```python
from build123d import *

# Parameters (mm, degrees)
F0_W     = 90
F0_H     = 41.77
F1_DEPTH = 6
F3_DEPTH = 36.63
F4_R     = 3
F5_R     = 1.5
F6_DEPTH = 5


with BuildPart() as f1:
    # F0 (on Front) → F1 (new body, symmetric)
    with BuildSketch(Plane.XZ):
        Rectangle(F0_W, F0_H)
    extrude(amount=F1_DEPTH, both=True)

    # F2 (on face) → F3 (join)
    with BuildSketch(Plane.XY.offset(20.885)):
        with BuildLine():
            Line((-28, 0), (-23, 0))
            ThreePointArc((-23, 0), (-28, 5), (-33, 0))
            Line((-33, 0), (-28, 0))
        make_face()
        with BuildLine():
            ThreePointArc((-33, 0), (-28, -5), (-23, 0))
            Line((-23, 0), (-28, 0))
            Line((-28, 0), (-33, 0))
        make_face()
        with BuildLine():
            Line((-5, 0), (0, 0))
            Line((0, 0), (5, 0))
            ThreePointArc((5, 0), (0, 5), (-5, 0))
        make_face()
        with BuildLine():
            Line((5, 0), (0, 0))
            Line((0, 0), (-5, 0))
            ThreePointArc((-5, 0), (0, -5), (5, 0))
        make_face()
        with BuildLine():
            ThreePointArc((33, 0), (28, 5), (23, 0))
            ThreePointArc((23, 0), (28, -5), (33, 0))
        make_face()
    extrude(amount=F3_DEPTH)

    # F4
    f4_edges = [f1.edges().sort_by_distance(p)[0] for p in [
        (45, -6, 0),
        (45, 6, 0),
        (-45, -6, 0),
        (-45, 6, 0),
    ]]
    fillet(f4_edges, radius=F4_R)

    # F5 (on face) → F6 (join)
    with BuildSketch(Plane.XY.offset(57.515)):
        with Locations((-28, 0)):
            Circle(F5_R)
        Circle(F5_R)
        with Locations((28, 0)):
            Circle(F5_R)
    extrude(amount=F6_DEPTH)


solid = f1.part
```
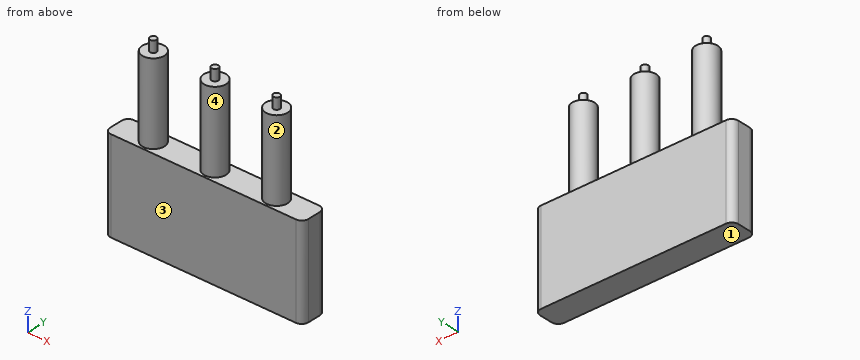
Can you work these out from the model? Positions are in its coordinate system, mm. Face numbers are marked on the shaded views. A direction names the side the tool comes from. Round coordinates to 2 decimals unless told otherwise and drop trailing zeros. Order: outer loops, then holes, each group sorted by start corner. A loop starts at its lowest first (then second) coordinate and runs counter-clockwise, first axis right, second up.
(1) If we section it at A-A (x = -28): Please give me the cut outline in (y, z) (3 decimals), plus the area to 3 significant figures.
Results are:
outline: (-6, -20.885) - (6, -20.885) - (6, 20.885) - (5, 20.885) - (5, 57.515) - (1.5, 57.515) - (1.5, 62.515) - (-1.5, 62.515) - (-1.5, 57.515) - (-5, 57.515) - (-5, 20.885) - (-6, 20.885) - close
area: 883 mm2
(2) If I drill on L1, parallel to X at y = -1, z = 39; L2, parallel to X at y = -4.5, z = 31; L3, parallel to Z at x = 15.5, y = -0.25 (3 decimals), over which ranges is the centre line in solid material (lowest first)?
Results are:
L1: x = -32.9 to -23.1, -4.9 to 4.9, 23.1 to 32.9
L2: x = -30.18 to -25.82, -2.18 to 2.18, 25.82 to 30.18
L3: z = -20.885 to 20.885
(3) If we section it at B-B (z = 25.5): Please give me the cut outline in (x, y).
Results are:
outline: circle Ø10 at (-28, 0); circle Ø10 at (0, 0); circle Ø10 at (28, 0)
(4) On a 3-axis mill with a long thin cutter (end or side, diameter ignored), from which of +Z, -Z, +X, -X, +Y, -Y can I reach the whole of each face in a straight line? I mean the marked faces 3 and 4. Say none if no direction works.
Results are:
face 3: +Z, -Z, +X, -X, -Y
face 4: +Z
(5) I'm going to push flat-ended pins straight in: pin 1 (4 mm diameter, centred on x = -23.5, z = 31.5, fed in from -Y); pin 2 (6 mm diameter, centred on y = -1.5, z = 40.5, fed in from -X); pin 3 (10 mm diameter, centred on x = 34.5, z = 36.5, fed in from -Y). Where does each tip first touch, or does it pass through?
Results are:
pin 1: stops at y = -4.33
pin 2: stops at x = -33
pin 3: stops at y = -4.77
(6) We'd pull the mould along X, two halves only. Please class the marked faces 1 and 2: +X half, -X half, draft (parallel to the pull), parting line (faces both ways), or undercut.
Results are:
face 1: draft
face 2: undercut
(7) If we section it at C-C (x = -10): Please give me the cut outline in (y, z) (3 decimals), plus the area to 3 significant figures.
Results are:
outline: (-6, -20.885) - (6, -20.885) - (6, 20.885) - (-6, 20.885) - close
area: 501 mm2
